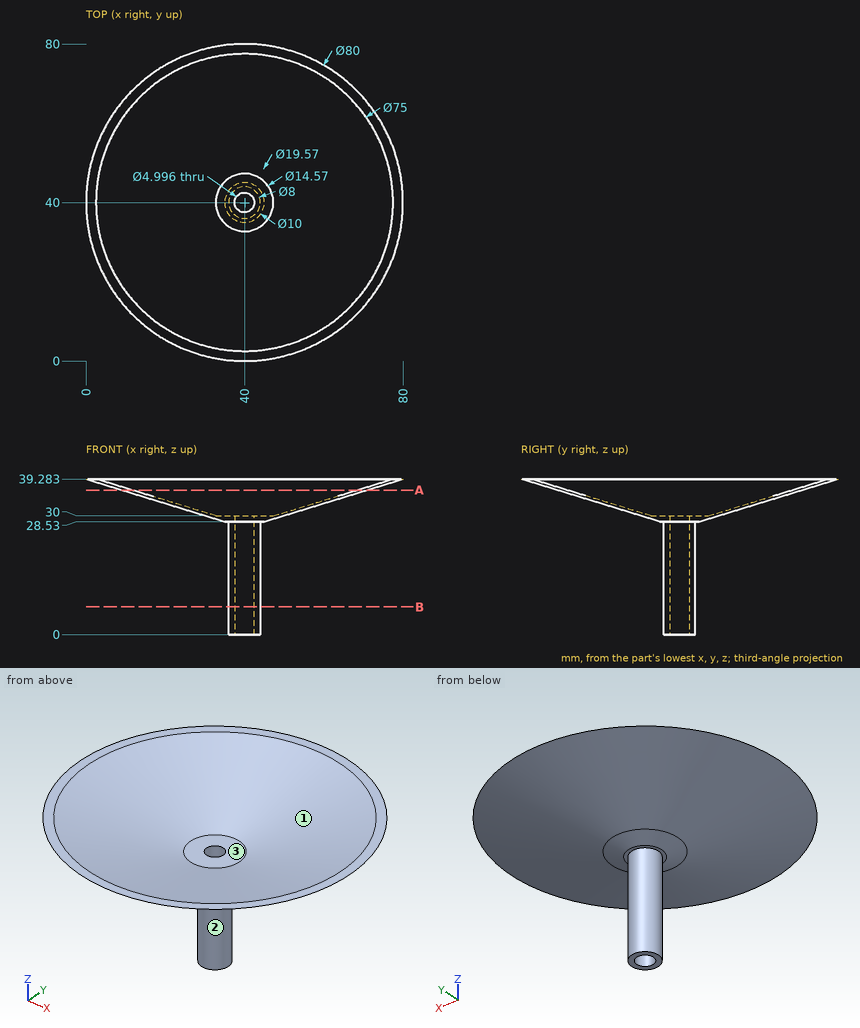
Here's the drawing with two shaded views (mm, measured from the low corner). I have some questions. Give positions to 0.01 mm unless a question says otherwise; leave off trailing zeros. Loops run counter-clockwise (first coordinate to the right, second up) from the corner with the lowest first, then second, coordinate; pieces in that order, holes last. Notation, with made-up numbers: M 4.25,-0.75 L 40.25,-0.75 A29 cw 40.25,23.25 Z; hole C 43.25,24 d4. An arc over 180 degrees is marked long. Use one line per item in the form item = value. Start each with the question number.
Q1. I need wall thicknesses on line 1 along Y through (x, z) = (40, 9.25); line 2 along Y through (x, z) = (38.5, 4.5); line 3 along Z through (x, y) = (30.5, 49.5). Which ranges of each line are inside material? Lowest first, please.
Q2. If we section it at A-A (z = 36.5): Write out the boundary of the cut face in (x, y).
Q3. Thinking about a two-plate mould opening in Y: for the marked faces 1, 2 and 3, which applies, +Y half, -Y half, draft (parallel to the pull), parting line (faces both ways), or undercut?
Q4. If we section it at B-B (z = 7): Write out the boundary of the cut face in (x, y).
Q5. Will these pins go through, and if not, where does the flat tip stop? pin 1 Ø8 at (x, y) = (40, 40) entering from -Z; pin 2 Ø7.5 at (x, y) = (39.5, 40) entering from +Z; pin 3 Ø1 at (x, y) = (34, 25.5) entering from -Z; pin 4 Ø10 at (x, y) = (71, 50.5) entering from -Z.
Taken from the geometry:
q1.line_1 = 36 to 37.5, 42.5 to 44
q1.line_2 = 36.29 to 38, 42 to 43.71
q1.line_3 = 31.12 to 31.89
q2.outline = C 40,40 d61.88; hole C 40,40 d56.88
q3.face_1 = undercut
q3.face_2 = parting line
q3.face_3 = undercut
q4.outline = C 40,40 d8; hole C 40,40 d5
q5.pin_1 = 0
q5.pin_2 = 30
q5.pin_3 = 31.66
q5.pin_4 = 35.51
